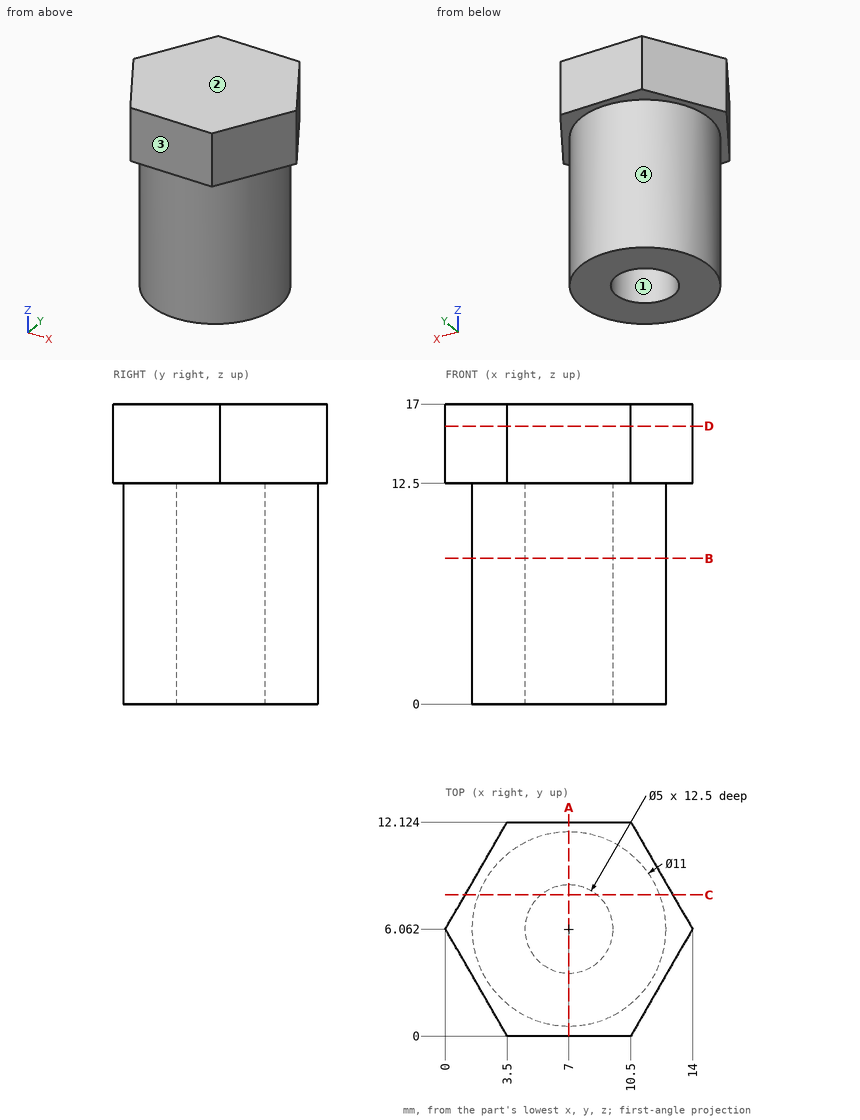
Input: dimensioned drawing with shaded views. Units: mm. Origin: part minimum x, y, z. Give positions to 0.01 mm unless a question says otherwise; leave off trailing zeros. Write each loop counter-clockwise with the first axis right and the second up, starting at its lowest first coordinate (ties: lowest second). Pieces come first, ordered by that corner, then holes. Notation, with made-up numbers: M 60.5,0.5 L 113.5,0.5 A18 ccw 113.5,6.5 Z; hole C 38.5,84 d7. An arc over 180 degrees is marked long. Return JSON: item names as keys, results as strings. Group by question number.
1) Cut plane B-B, the plane z = 8.25. Output: boundary loops of the cut face in (x, y), plus the area to 3 significant figures.
2) Pull-direction query (Y, two-part tool) for the marked faces 1, 2, 3 and 4; classes: pulls with the +Y half, pulls with the -Y half, needs draft (parallel to the pull), parting line crosses it, or undercut.
3) Cut plane D-D, the plane z = 15.75. Output: boundary loops of the cut face in (x, y) (1 decimal).
4) Cut plane C-C, the plane y = 8. Output: boundary loops of the cut face in (x, z), plus the area to 3 significant figures.
5) Pin query (flat end, axial travel): P1, Ø4, axis at y = 2.5, z = 7, coming from the +X side; P2, Ø1.5, axis at x = 9, z = 8.5, coming from the +Y side; P3, Ø1.5, axis at x = 7, y = 5.5, coming from the -Z side. Return the tip coordinate at first contact, or that it passes through.
6) Cut plane A-A, the plane x = 7. Output: boundary loops of the cut face in (y, z) (1 decimal).
7) Material intervals for line 1 along Y through (x, z) = (7, 3.75); line 2 along Y through (x, z) = (7.5, 6.75) (1 decimal); line 3 along X through (y, z) = (8, 6.75) (1 decimal), sorted ascending. Write a range as [from, to].
Recorded:
{
 "1": {"outline": "C 7,6.06 d11; hole C 7,6.06 d5", "area": "75.4 mm²"},
 "2": {"face 1": "undercut", "face 2": "needs draft", "face 3": "pulls with the -Y half", "face 4": "parting line crosses it"},
 "3": {"outline": "M 0,6.1 L 3.5,0 L 10.5,0 L 14,6.1 L 10.5,12.1 L 3.5,12.1 Z"},
 "4": {"outline": "M 1.12,12.5 L 1.85,12.5 L 1.85,0 L 5.42,0 L 5.42,12.5 L 8.58,12.5 L 8.58,0 L 12.15,0 L 12.15,12.5 L 12.88,12.5 L 12.88,17 L 1.12,17 Z", "area": "142 mm²"},
 "5": {"P1": "stops at x = 12.27", "P2": "stops at y = 11.42", "P3": "stops at z = 12.5"},
 "6": {"outline": "M 0,12.5 L 0.6,12.5 L 0.6,0 L 3.6,0 L 3.6,12.5 L 8.6,12.5 L 8.6,0 L 11.6,0 L 11.6,12.5 L 12.1,12.5 L 12.1,17 L 0,17 Z"},
 "7": {"line 1": "y = [0.56, 3.56], [8.56, 11.56]", "line 2": "y = [0.6, 3.6], [8.5, 11.5]", "line 3": "x = [1.9, 5.4], [8.6, 12.1]"}
}
